Source: CAD feature listing. Evaluate the final solid. Frame: model axes, mm. A direction names the side the tool comes from. Coordinates: 2 decimals unless noted, no trailing zeros. Loops run counter-clockwise (first coordinate to the right, second up) from the corner with the lowest first, then second, coordinate; pieces in that order, holes last. Notation, with made-up numbers: (79.5, 69.5) -> (128.5, 69.5) arc R31 cw to (128.5, 104.5) -> close; hole circle Ø4 at (-12.5, 65). An arc over 180 degrees is marked (long way). Answer as a JSON object with one key per item and string values. Group by question number.
from build123d import *

# Parameters (mm, degrees)
CHANFREIN1_SIZE = 0.5


with BuildPart() as part:
    # Esquisse1 → Base-Révolution (revolve)
    with BuildSketch(Plane.XY, mode=Mode.PRIVATE) as base_r_volution_sk:
        Polygon((0, 28), (6, 28), (6, 26), (4, 26), (4, 24), (3.5, 24), (3.5, 12), (3, 12), (3, 0), (0, 0), align=None)
    revolve(base_r_volution_sk.sketch.rotate(Axis((0, 0, 0), (0, 1, 0)), 90), axis=Axis((0, 0, 0), (0, 1, 0)))

    # Chanfrein1
    chanfrein1_edges = [part.edges().sort_by_distance(p)[0] for p in [
        (0, 28, 6),
        (0, 0, 3),
    ]]
    chamfer(chanfrein1_edges, length=CHANFREIN1_SIZE)

    # Esquisse3 → Enlever de la matière-Révolution1 (revolve, cut)
    with BuildSketch(Plane(origin=(0, 0, 0), x_dir=(0, 0, -1), z_dir=(1, 0, 0))):
        with BuildLine():
            Line((2.25, 12), (3, 12))
            Line((3, 12), (3, 10.5))
            Line((3, 10.5), (2.25, 10.5))
            ThreePointArc((2.25, 10.5), (1.5, 11.25), (2.25, 12))
        make_face()
    revolve(axis=Axis((0, 0, 0), (0, 1, 0)), mode=Mode.SUBTRACT)


solid = part.part
1. Pin query (flat end, axial travel): pin 1 Ø1.5 at (x, y) = (-3.5, 11.5) entering from -Z; pin 2 Ø4 at (y, z) = (23.5, -1.5) entering from -X; pin 3 Ø1.5 at (y, z) = (9.5, -4) entering from +X; pin 4 Ø4 at (x, y) = (4, 13.5) entering from -Z. Return the tip coordinate at first contact, or that it passes through.
2. Section query D-D on y = 19. Return loops of the section in (x, z), then the cut area to 3 significant figures.
3. Reachability of faces 1 (the face through (0.7, 12, -2.3)), 2 (the face through (3.905, 24.986, 0.867)), 3 (the face through (0, 28, 0)) from +Z, -Z, +X, -X, +Y, -Y: full face, straight path, thin tool, end or side. Return the list, or none.
4. Ray query, L1, parallel to Y at x = -1.75, z = 1.25; L2, parallel to Y at x = -1.5, z = 4; L3, parallel to Y at x = -1.5, z = -3. Return the intervals inside material, ascending.
5. Section query A-A on z = 0. Return loops of the section in (x, y).
6. Section query B-B on x = 0. Return loops of the section in (y, z), then the cut area to 3 significant figures.
7. Section query C-C on y = 7. Return loops of the section in (x, z), then the cut area to 3 significant figures.
Solved:
{
 "1": {"pin 1": "z = -1.9", "pin 2": "x = -4", "pin 3": "through", "pin 4": "z = -2.87"},
 "2": {"outline": "circle Ø7 at (0, 0)", "area": "38.5 mm^2"},
 "3": {"face 1": "none", "face 2": "-Y", "face 3": "+Z, -Z, +X, -X, +Y"},
 "4": {"L1": "0 to 10.51, 11.99 to 28", "L2": "26 to 28", "L3": "12 to 28"},
 "5": {"outline": "(-6, 26) -> (-4, 26) -> (-4, 24) -> (-3.5, 24) -> (-3.5, 12) -> (-2.25, 12) arc R0.75 cw to (-2.25, 10.5) -> (-3, 10.5) -> (-3, 0.5) -> (-2.5, 0) -> (2.5, 0) -> (3, 0.5) -> (3, 10.5) -> (2.25, 10.5) arc R0.75 cw to (2.25, 12) -> (3.5, 12) -> (3.5, 24) -> (4, 24) -> (4, 26) -> (6, 26) -> (6, 27.5) -> (5.5, 28) -> (-5.5, 28) -> (-6, 27.5) -> close"},
 "6": {"outline": "(0, -2.5) -> (0.5, -3) -> (10.5, -3) -> (10.5, -2.25) arc R0.75 cw to (12, -2.25) -> (12, -3.5) -> (24, -3.5) -> (24, -4) -> (26, -4) -> (26, -6) -> (27.5, -6) -> (28, -5.5) -> (28, 5.5) -> (27.5, 6) -> (26, 6) -> (26, 4) -> (24, 4) -> (24, 3.5) -> (12, 3.5) -> (12, 2.25) arc R0.75 cw to (10.5, 2.25) -> (10.5, 3) -> (0.5, 3) -> (0, 2.5) -> close", "area": "191 mm^2"},
 "7": {"outline": "circle Ø6 at (0, 0)", "area": "28.3 mm^2"}
}
